```python
from build123d import *

# Parameters (mm, degrees)
F0_R     = 0.625
F1_DEPTH = 25


with BuildPart() as f1:
    # F0 (on Top) → F1 (new body)
    with BuildSketch(Plane.XY):
        with BuildLine():
            Line((-84.169807, 17.273173), (-78.204214, 17.272388))
            ThreePointArc((-78.204214, 17.272388), (-77.454115, 18.022352), (-78.204142, 18.772388))
            Line((-78.204142, 18.772388), (-80.222164, 18.772315))
            Line((-80.222164, 18.772315), (-80.222146, 18.272315))
            Line((-80.222146, 18.272315), (-82.222146, 18.272243))
            Line((-82.222146, 18.272243), (-82.222164, 18.772243))
            Line((-82.222164, 18.772243), (-84.18612, 18.772172))
            Line((-84.18612, 18.772172), (-84.222164, 18.772171))
            ThreePointArc((-84.222164, 18.772171), (-84.95407, 18.030621), (-84.23862, 17.273182))
            Line((-84.23862, 17.273182), (-84.169807, 17.273173))
        make_face()
        with Locations((-84.204115, 18.022388)):
            Circle(F0_R, mode=Mode.SUBTRACT)
        with Locations((-78.204115, 18.022388)):
            Circle(F0_R, mode=Mode.SUBTRACT)
        with BuildLine():
            ThreePointArc((-84.23862, 17.273182), (-84.204214, 17.272388), (-84.169807, 17.273173))
            Line((-84.169807, 17.273173), (-84.23862, 17.273182))
        make_face()
        with BuildLine():
            ThreePointArc((-84.18612, 18.772172), (-84.204142, 18.772388), (-84.222164, 18.772171))
            Line((-84.222164, 18.772171), (-84.18612, 18.772172))
        make_face()
    extrude(amount=F1_DEPTH)


solid = f1.part
```
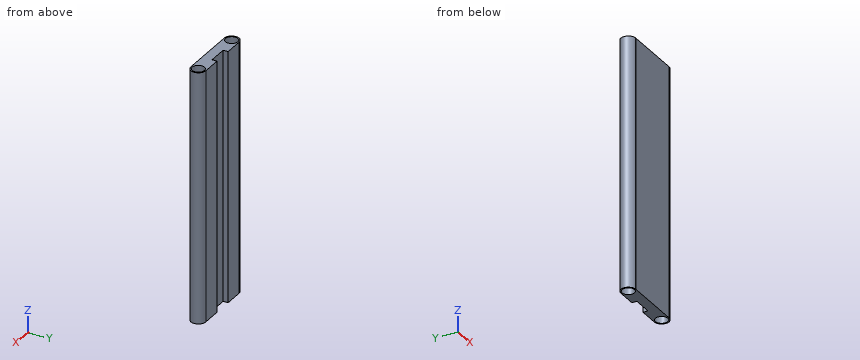
Verification items for the finished model (mm, model axes). Round coordinates to 2 decimals unless told otherwise and drop trailing zeros. Order: outer loops, then holes, each group sorted by start corner. A loop starts at its lowest first (then second) coordinate and runs counter-clockwise, first axis right, second up. Notation, with made-up numbers: (47.25, 36.5) -> (73.25, 36.5) arc R20 cw to (73.25, 51.5) -> close; hole circle Ø8 at (6, 23.25). An arc over 180 degrees is marked (long way). Put each result on its own line as item: value. Start each with the question number.
(1) Section check B-B (z = 9). State how many separate pieces and enclosed holes the cut face has, then the cut area to 3 significant figures.
(2) Material ranges on line 1 along X through (y, z) = (18.5, 11.5); line 2 along X through (y, z) = (18.45, 4); line 3 along X through (y, z) = (18.7, 10.5), recorded low to high.
(3) Depth check by flat-ended pin: pin 1 Ø0.6 at (x, z) = (-81, 14) entering from +Y. Enter the tip coordinate at first touch or a pass-through.
(4) Section check A-A (y = 17.75). Enter the section's corners in (x, z).
Completed:
1. separate pieces: 1
1. enclosed holes: 2
1. area: 7.31 mm2
2. line 1: x = -84.78 to -84.61, -83.8 to -82.22, -80.22 to -78.61, -77.8 to -77.63
2. line 2: x = -84.82 to -84.66, -83.75 to -82.22, -80.22 to -78.66, -77.75 to -77.59
2. line 3: x = -84.53 to -82.22, -80.22 to -77.88
3. pin 1: stops at y = 18.27
4. outline: (-84.9, 0) -> (-84.77, 0) -> (-84.77, 25) -> (-84.9, 25) -> close; (-83.64, 0) -> (-78.77, 0) -> (-78.77, 25) -> (-83.64, 25) -> close; (-77.64, 0) -> (-77.51, 0) -> (-77.51, 25) -> (-77.64, 25) -> close
